Source: CAD feature listing. Evaluate the final solid. Frame: model axes, mm. Face numbers are marked on the shaded views. A direction names the side the tool comes from. Round coordinates to 2 decimals unless told otherwise and drop trailing zeros. Loops run counter-clockwise (first coordinate to the right, second up) from the corner with the lowest first, then second, coordinate; pieces in that order, holes last. Notation, with made-up numbers: (35, -13.75) -> (71, -13.75) arc R20 cw to (71, -6.75) -> close; hole circle Ø1 at (41, 43.5). An arc over 180 degrees is marked (long way). Put each result on its own line as item: value. Start each with the question number.
1. Draft query along Y for the marked faces 1, 2, 3 and 4. Return one class per face: pulls with the +Y half, pulls with the -Y half, needs draft (parallel to the pull), parting line crosses it, or undercut.
2. Contact query for flat-ended pins moving along their axis: pin 1 (2.5 mm diameter, centred on x = -5.5, z = 9, fed in from -Y); pin 2 (5 mm diameter, centred on x = 6, z = 3, fed in from +Y); pin 3 (3.5 mm diameter, centred on x = 6.5, z = 8.5, fed in from +Y); pin 4 (2.5 mm diameter, centred on x = 8.84, y = 5.3, fed in from +Z). Output: stop coordinate, or through.
3. Cut plane A-A (y = -12). Return the cut outline in (x, z).
4. Set-up query: the marked faces 5, 6 and 7. Return all of +Z, -Z, +X, -X, +Y, -Y with unobstructed straight access to the full face (end or side cutting, diameter ignored); none if empty.
5. Cut plane D-D (x = -11). Return the cut outline in (y, z).
6. Cut plane B-B (z = 8.75). State how many separate pieces and enclosed holes the cut face has, then the cut area to 3 significant figures.
7. Material intervals for L1, parallel to Y at x = 5, z = 7.75; L2, parallel to Y at x = 8, z = 0.5; L3, parallel to X at y = 4.5, z = 5.75, sorted ascending.
```python
from build123d import *

# Parameters (mm, degrees)
SKETCH2_R           = 15
BOSS_EXTRUDE1_DEPTH = 10
CUT_EXTRUDE1_DEPTH  = 4
FILLET1_R           = 1
SKETCH4_R           = 1
CUT_EXTRUDE2_DEPTH  = 10
CIRPATTERN1_COUNT   = 4


with BuildPart() as part:
    # Sketch2 → Boss-Extrude1 (new body)
    with BuildSketch(Plane.XY):
        Circle(SKETCH2_R)
    extrude(amount=BOSS_EXTRUDE1_DEPTH)

    # Sketch3 → Cut-Extrude1 (cut)
    with BuildSketch(Plane.XY.offset(10)):
        Polygon((-1.25, 1.25), (-1.25, 15.296025934), (1.25, 15.296025934), (1.25, 1.25), (15.674686846, 1.25), (15.674686846, -1.25), (1.25, -1.25), (1.25, -15.629214974), (-1.25, -15.629214974), (-1.25, -1.25), (-15.410512851, -1.25), (-15.410512851, 1.25), align=None)
    extrude(amount=-CUT_EXTRUDE1_DEPTH, mode=Mode.SUBTRACT)

    # Fillet1
    fillet1_edges = [part.edges().sort_by_distance(p)[0] for p in [
        (-8.098912964, 1.25, 6),
        (-1.25, 8.098912964, 6),
        (1.25, 8.098912964, 6),
        (8.098912964, 1.25, 6),
        (8.098912964, -1.25, 6),
        (1.25, -8.098912964, 6),
        (-1.25, -8.098912964, 6),
        (-8.098912964, -1.25, 6),
    ]]
    fillet(fillet1_edges, radius=FILLET1_R)

    # Sketch4 → Cut-Extrude2 (cut)
    with BuildSketch(Plane.XY.offset(10)):
        with Locations((-5.303300859, 8.838834765)):
            Circle(SKETCH4_R)
        with Locations((-8.838834765, 5.303300859)):
            Circle(SKETCH4_R)
    cut_extrude2 = extrude(amount=-CUT_EXTRUDE2_DEPTH, mode=Mode.SUBTRACT)

    # CirPattern1: Cut-Extrude2 ×4 about axis
    cirpattern1_axis = Axis((0, 0, 0), (0, 0, 1))
    for i in range(1, CIRPATTERN1_COUNT):
        add(cut_extrude2.rotate(cirpattern1_axis, i * 360 / CIRPATTERN1_COUNT), mode=Mode.SUBTRACT)


solid = part.part
```
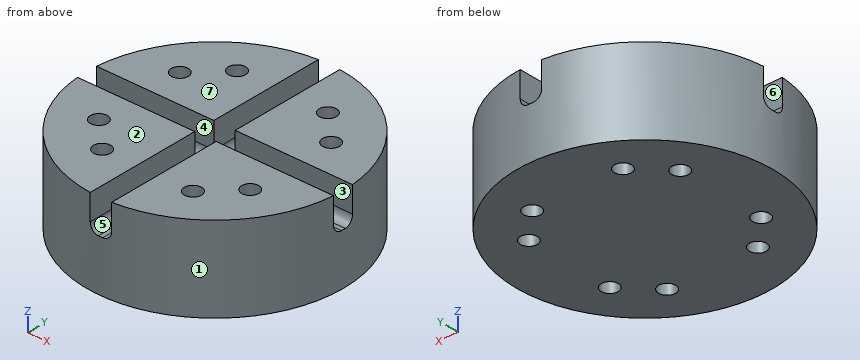
Solution:
1. face 1: parting line crosses it
1. face 2: needs draft
1. face 3: undercut
1. face 4: undercut
2. pin 1: stops at y = -14.39
2. pin 2: stops at y = 14.59
2. pin 3: stops at y = 14.23
2. pin 4: stops at z = 10
3. outline: (-9, 0) -> (9, 0) -> (9, 10) -> (1.25, 10) -> (1.25, 7) arc R1 cw to (0.25, 6) -> (-0.25, 6) arc R1 cw to (-1.25, 7) -> (-1.25, 10) -> (-9, 10) -> close
4. face 5: +Z, +Y, -Y
4. face 6: +Z, +X, -X
4. face 7: +Z, +X, -X, +Y, -Y
5. outline: (-10.2, 0) -> (10.2, 0) -> (10.2, 10) -> (1.25, 10) -> (1.25, 7) arc R1 cw to (0.25, 6) -> (-0.25, 6) arc R1 cw to (-1.25, 7) -> (-1.25, 10) -> (-10.2, 10) -> close
6. separate pieces: 4
6. enclosed holes: 8
6. area: 538 mm^2
7. L1: y = -14.14 to -9.79, -7.89 to -1.25, 1.25 to 7.89, 9.79 to 14.14
7. L2: y = -12.69 to -5.85, -4.76 to 4.76, 5.85 to 12.69
7. L3: x = -14.31 to -9.43, -8.24 to 8.24, 9.43 to 14.31
